Study the drawing (mm; zero at the part's minimum x, y, z) and answer. Coordinates: 2 decimals unless noted, no trailing zeros. Order: outer loops, then holes, each group sorted by start corner. A loop starts at its lowest first (then second) coordinate and runs counter-clockwise, first axis right, second up.
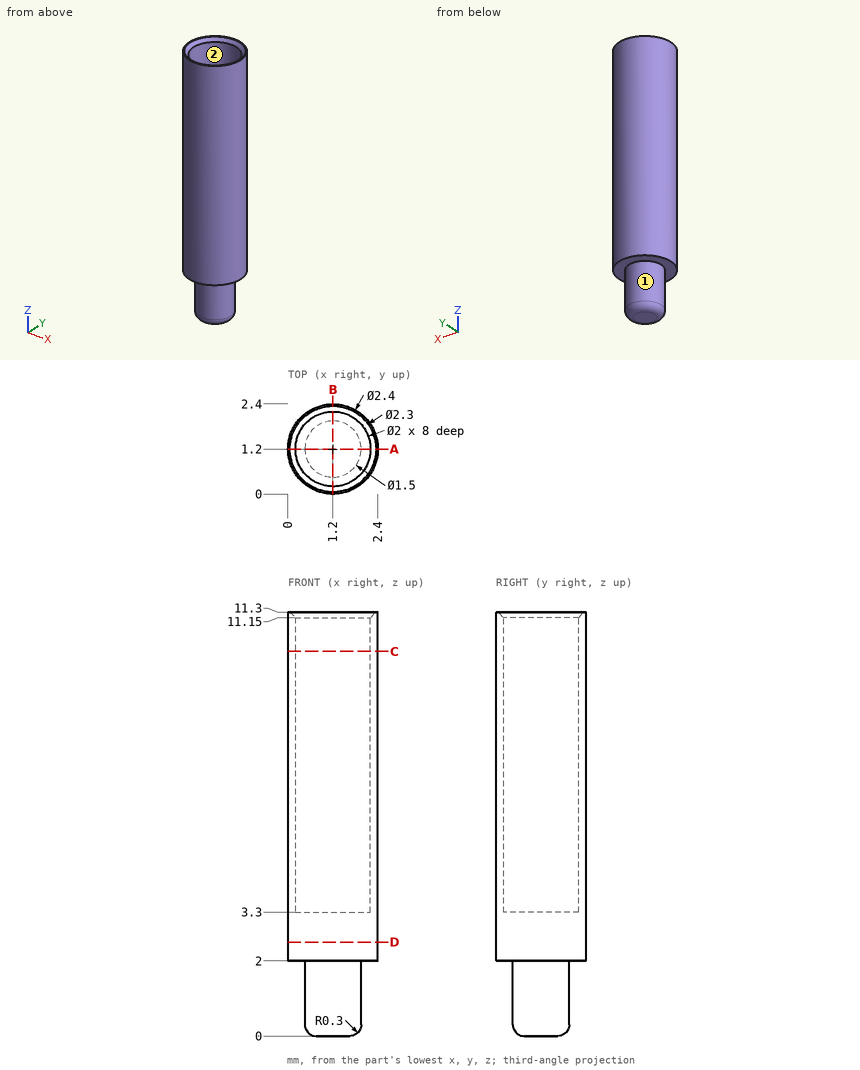
1) A cutting plane is placed at D-D, the plane z = 2.5. Determine the outline of the cut face in (x, y), and give its area (3 significant figures).
A:
outline: circle Ø2.4 at (1.2, 1.2)
area: 4.52 mm2
2) Determine the mould class of the marked faces 1 and 2 for opening direction Y: pulls with the +Y half, pulls with the -Y half, needs draft (parallel to the pull), parting line crosses it, or undercut.
A:
face 1: parting line crosses it
face 2: undercut
3) A cutting plane is placed at C-C, the plane z = 10.25. Determine the outline of the cut face in (x, y), and give its area (3 significant figures).
A:
outline: circle Ø2.4 at (1.2, 1.2); hole circle Ø2 at (1.2, 1.2)
area: 1.38 mm2
4) Straight lines are drawn through the part: line 1 (Y direction, x = 1.2, z = 5.5); line 2 (Z direction, x = 1.3, y = 1.25); line 3 (Y direction, x = 1.75, z = 9.25). For each, find the intervals that lie inside material, in ascending order.
A:
line 1: y = 0 to 0.2, 2.2 to 2.4
line 2: z = 0 to 3.3
line 3: y = 0.13 to 0.36, 2.04 to 2.27
5) A cutting plane is placed at A-A, the plane y = 1.2. Determine the outline of the cut face in (x, z), and give its area (3 significant figures).
A:
outline: (0, 2) - (0.45, 2) - (0.45, 0.3) arc R0.3 ccw to (0.75, 0) - (1.65, 0) arc R0.3 ccw to (1.95, 0.3) - (1.95, 2) - (2.4, 2) - (2.4, 11.3) - (2.35, 11.3) - (2.2, 11.15) - (2.2, 3.3) - (0.2, 3.3) - (0.2, 11.15) - (0.05, 11.3) - (0, 11.3) - close
area: 9.26 mm2
6) A flat-ended cylindrical pin translates along its axis: pin 1 Ø1 at (x, z) = (0.5, 5.5) entering from -Y. Find the tip coordinate at first contact, or state that the pin passes through.
A:
pin 1: stops at y = 0.02
